Work out the finished part from the listing and answer in its coordinate system (mm). Give positions to 0.01 mm unless a question says otherwise; leave off trailing zeros. Order: outer loops, then holes, each group sorted by start corner. A loop starts at its lowest first (then second) coordinate and runs counter-clockwise, first axis right, second up. Notation, with made-up numbers: (3.25, 72.5) -> (7.25, 72.5) arc R34 cw to (7.25, 102.5) -> close; hole circle Ø9 at (54.25, 86.5). An arc over 180 degrees is marked (long way). Use a Markdown table: item, result. Add a question column.
```python
from build123d import *

# Parameters (mm, degrees)
F0_W     = 57.15
F0_H     = 31.75
F1_DEPTH = 25.4
F3_DEPTH = 25.4
F5_DEPTH = 25.4


with BuildPart() as f1:
    # F0 (on Front) → F1 (new body)
    with BuildSketch(Plane.XZ):
        with Locations((-7.4283964932, 25.9043908785)):
            Rectangle(F0_W, F0_H)
    extrude(amount=F1_DEPTH)

    # F2 (on face) → F3 (cut)
    with BuildSketch(Plane.XZ.offset(25.4)):
        with BuildLine():
            ThreePointArc((2.0966035068, 41.7793908785), (9.2454078798, 31.865097438), (21.1466035068, 29.0793908785))
            Line((21.1466035068, 29.0793908785), (21.1466035068, 41.7793908785))
            Line((21.1466035068, 41.7793908785), (2.0966035068, 41.7793908785))
        make_face()
    extrude(amount=-F3_DEPTH, mode=Mode.SUBTRACT)

    # F4 (on face) → F5 (cut)
    with BuildSketch(Plane.XZ.offset(25.4)):
        with BuildLine():
            Line((-36.0033964932, 41.7793908785), (-36.0033964932, 35.4293908785))
            Line((-36.0033964932, 35.4293908785), (-36.0033964932, 29.0793908785))
            ThreePointArc((-36.0033964932, 29.0793908785), (-32.2836526143, 38.0596469995), (-23.3033964932, 41.7793908785))
            Line((-23.3033964932, 41.7793908785), (-36.0033964932, 41.7793908785))
        make_face()
    extrude(amount=-F5_DEPTH, mode=Mode.SUBTRACT)


solid = f1.part
```
1) The part is cut by section C-C, the plane z = 30.5. Determine the outline of the cut face in (x, y), then the cut area to 3 significant figures.
2) A flat-ended cylindrical pin translates along its axis: pin 1 (5 mm diameter, centred on y = -9, z = 36.5, fed in from +X). Find the tip coordinate at first contact, or state that the pin passes through.
3) The part is cut by section A-A, the plane y = -14. Determine the outline of the cut face in (x, z), then the cut area to 3 significant figures.
4) The part is cut by section B-B, the plane x = -28. Determine the outline of the cut face in (y, z).
5) Determine the mould class of faces 1 (the cylindrical face through (-32.38, -12.88, 37.96)), 2 (the flat face through (-11, -13, 41.779)), 3 (the cylindrical face through (9.1, -12.878, 31.963)) for opening direction X: released by +X, released by -X, zero draft, split by the parting line, or undercut.
6) Straight lines are drawn through the part: line 1 (Z direction, x = -23.5, y = -17.25); line 2 (X direction, y = -18.25, z = 38.5); line 3 (Z direction, x = -25, y = -19.75). For each, find the intervals that lie inside material, in ascending order.
A:
| question | item | result |
|---|---|---|
| 1 | outline | (-35.92, -25.4) -> (11.7, -25.4) -> (11.7, 0) -> (-35.92, 0) -> close |
| 1 | area | 1,210 mm^2 |
| 2 | pin 1 | x = 6.63 |
| 3 | outline | (-36, 10.03) -> (21.15, 10.03) -> (21.15, 29.08) arc R17.44 cw to (2.1, 41.78) -> (-23.3, 41.78) arc R12.7 ccw to (-36, 29.08) -> close |
| 3 | area | 1,590 mm^2 |
| 4 | outline | (-25.4, 10.03) -> (0, 10.03) -> (0, 40.88) -> (-25.4, 40.88) -> close |
| 5 | face 1 | released by -X |
| 5 | face 2 | zero draft |
| 5 | face 3 | undercut |
| 6 | line 1 | 10.03 to 41.78 |
| 6 | line 2 | -31.82 to 3.36 |
| 6 | line 3 | 10.03 to 41.67 |
